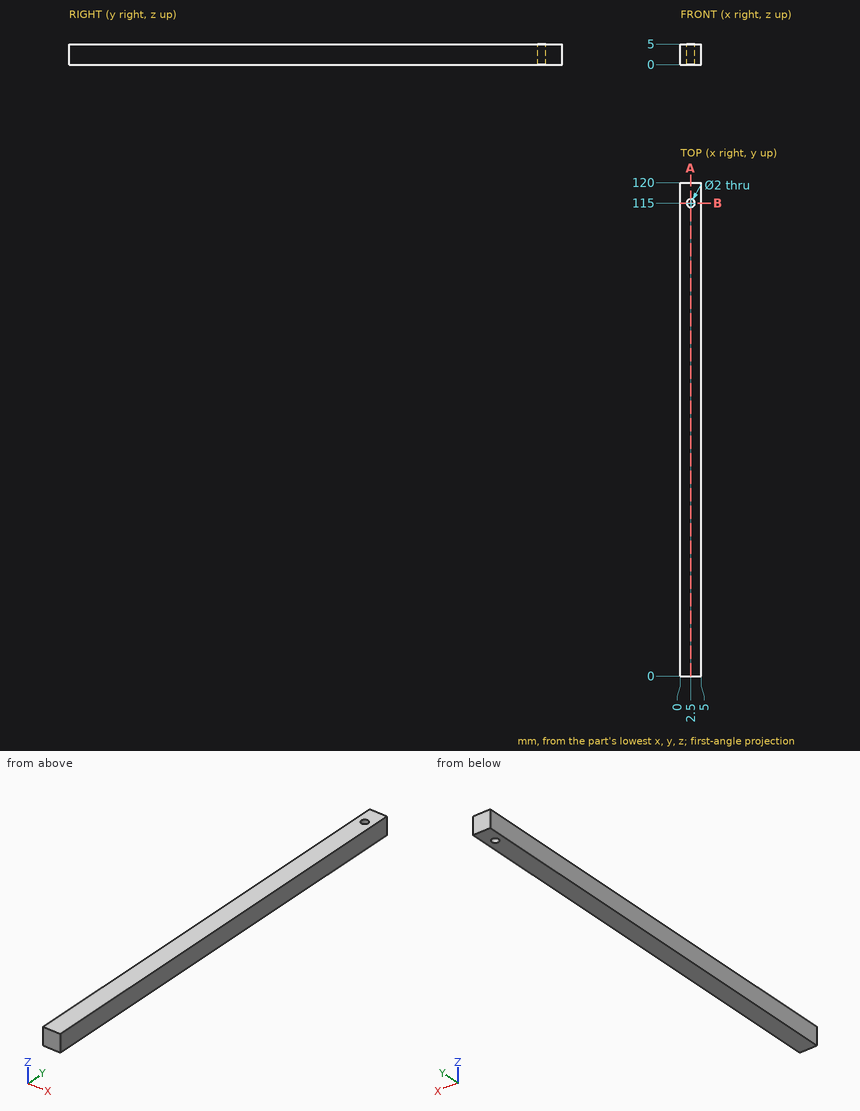
Input: dimensioned drawing with shaded views. Units: mm. Origin: part minimum x, y, z. Coordinates: 2 decimals unless noted, no trailing zeros. Loops run counter-clockwise (first coordinate to the right, second up) from the corner with the lowest first, then second, coordinate; pieces in that order, holes last. Notation, with made-up numbers: M -25.5,65 L 28.5,65 A15 cw 28.5,90 Z; hole C 43,40 d7. An arc over 180 degrees is marked long. One line per item, written item: value. Start each with the question number.
1) Cut plane A-A (x = 2.5). Return loops of the section in (y, z).
2) Cut plane B-B (y = 115). Return loops of the section in (x, z).
3) Pin query (flat end, axial travel): P1, Ø1.6, axis at x = 2.5, y = 115, coming from the +Z side; P2, Ø2, axis at y = 18, z = 1, coming from the -X side. Return the tip coordinate at first contact, or that it passes through.
4) Material intervals for L1, parallel to Y at x = 2.55, z = 1.55; L2, parallel to X at y = 115, z = 2; L3, parallel to Y at x = 1.65, z = 2.8, sorted ascending. Write a range as from..to.
Evaluation:
1. outline: M 0,0 L 114,0 L 114,5 L 0,5 Z; M 116,0 L 120,0 L 120,5 L 116,5 Z
2. outline: M 0,0 L 1.5,0 L 1.5,5 L 0,5 Z; M 3.5,0 L 5,0 L 5,5 L 3.5,5 Z
3. P1: through
3. P2: x = 0
4. L1: 0..114, 116..120
4. L2: 0..1.5, 3.5..5
4. L3: 0..114.47, 115.53..120
